Job drawing, mm, ordinate dimensions from the low corner. One solid piece. Round coordinates to 2 decimals unless told otherwise and drop trailing zeros. Write each loop counter-clockwise with the first axis right and the second up, starting at its lowest first coordinate (ties: lowest second). Pieces come first, ordered by that corner, then holes.
1) Saw through at D-D (y = 19). Write the cut outline in (x, z).
2) Pull direction X, two halves, no side cores. Call the marked faces 1, 2, 3 and 4: +X half, -X half, draft (parallel to the pull), parting line (faces both ways), or undercut.
3) Flat gauge pin, fed straight in: pin 1 (2 mm diameter, centred on y = 12, z = 2, fed in from +X) (1 decimal). Where does the tip first touch, or does it go through?
4) Saw through at C-C (x = 8). Write the cut outline in (y, z), plus the area to 3 significant figures.
5) Saw through at B-B (y = 12.65). Write the cut outline in (x, z).
6) Wall check: probe 1 along X at (y, z) = (14.25, 1.6) (1 decimal); probe 2 along X at (y, z) = (13.5, 2.6) (1 decimal); probe 3 along X at (y, z) = (16.75, 1.85) (1 decimal). Give the ranges that are in metal, low to high.
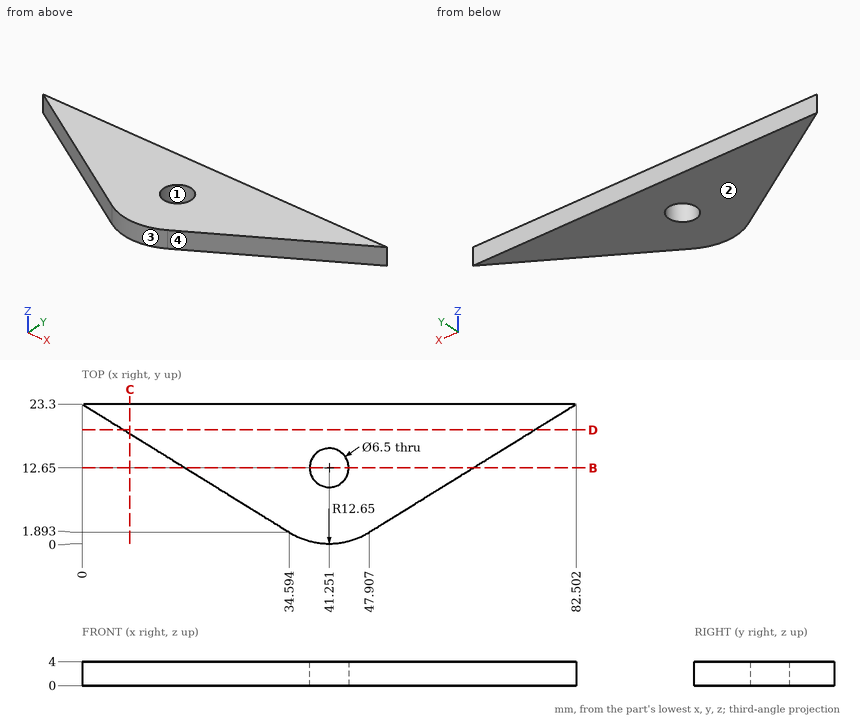
Evaluation:
1. outline: (6.95, 0) - (75.55, 0) - (75.55, 4) - (6.95, 4) - close
2. face 1: undercut
2. face 2: draft
2. face 3: parting line
2. face 4: +X half
3. pin 1: stops at x = 65.9
4. outline: (18.35, 0) - (23.3, 0) - (23.3, 4) - (18.35, 4) - close
4. area: 19.8 mm2
5. outline: (17.21, 0) - (38, 0) - (38, 4) - (17.21, 4) - close; (44.5, 0) - (65.29, 0) - (65.29, 4) - (44.5, 4) - close
6. probe 1: x = 14.6 to 38.4, 44.1 to 67.9
6. probe 2: x = 15.8 to 38.1, 44.4 to 66.7
6. probe 3: x = 10.6 to 71.9
